Part model, mm, in its own coordinate system. Face numbers are marked on the shaded views. A direction names the side the tool comes from. Coordinates: 2 decimals unless noted, no trailing zeros. Write each loop counter-clockwise with the first axis right and the second up, starting at its lowest first coordinate (ties: lowest second). Pieces come first, ordered by that corner, then holes. Notation, with made-up numbers: M 74,53.25 L 104,53.25 A20 ccw 104,65.25 Z; hole C -14,-10.75 d5. An arc over 180 degrees is marked long. Use a Markdown table: item, result. Add a question column.
Q1. Slice it at C-C on x = -3. Write the cut outline in (y, z), then the cut area to 3 significant figures.
Q2. Wall check: L1, parallel to Z at x = -1, y = 0.75; L2, parallel to Z at x = -2.5, y = 2.6; L3, parallel to X at y = 0.8, z = 6.75. Give the ranges that are in metal, low to high. Write a range as from..to.
Q3. Slice it at D-D on x = 0.75. Write the cut outline in (y, z).
Q4. Mould opens along Z. For the marked faces 3, 4 and 5 say: released by +Z, released by -Z, zero draft, split by the parting line, or undercut.
Q5. Slice it at B-B on y = 2.5. Write the cut outline in (x, z), then the cut area to 3 significant figures.
Q6. Tool access for the marked faces 1 and 2: list every direction of +Z, -Z, +X, -X, +Y, -Y with a clear straight run to the whole face (end or side of a thin tool).
Q7. Pin check, flat tip, straight feed: pin 1 Ø1.8 at (x, z) = (-2.04, 16.65) entering from +Y. Stop position of the tip, or through.
Q8. Slice it at A-A on z = 5.5. Write the cut outline in (x, y), then the cut area to 3 significant figures.
from build123d import *

# Parameters (mm, degrees)
SKETCH1_R           = 1.502144761
SKETCH1_R_2         = 1.500235367
BOSS_EXTRUDE3_DEPTH = 3


with BuildPart() as part:
    # Sketch1 → Boss-Extrude3 (new body)
    with BuildSketch(Plane(origin=(0, 0, 0), x_dir=(1, 0, 0), z_dir=(0, 1, 0))):
        Polygon((-3.272270882, -0.800771607), (-2.124220585, 1.970866991), (-1.964220585, 1.970866991), (-0.816170288, -0.800771607), (1.95546831, 0.34727869), (1.95546831, -17.15272131), (1.95546831, -19.653488119), (-6.043909479, -19.653488119), (-6.043909479, -17.27772131), (-6.043909479, -4.77772131), (-6.043909479, 0.34727869), align=None)
        with Locations((-2.04453169, -6.653488119)):
            Circle(SKETCH1_R, mode=Mode.SUBTRACT)
        with Locations((-2.04453169, -16.653488119)):
            Circle(SKETCH1_R_2, mode=Mode.SUBTRACT)
    extrude(amount=BOSS_EXTRUDE3_DEPTH)


solid = part.part
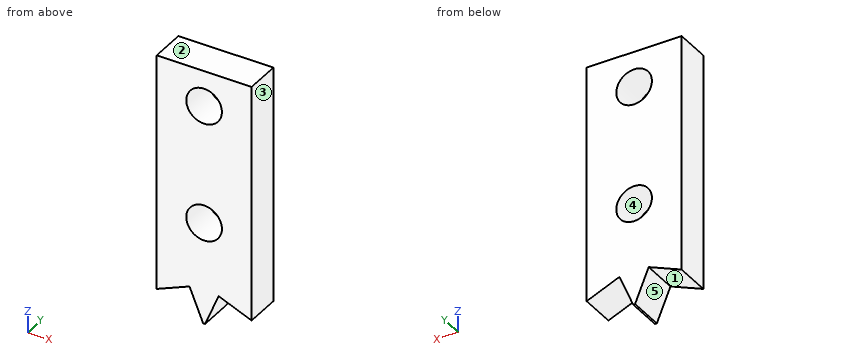
Recorded:
| question | item | result |
|---|---|---|
| 1 | outline | M 0,0.14 L 3,0.14 L 3,5.49 L 0,5.49 Z; M 0,7.81 L 3,7.81 L 3,15.5 L 0,15.5 Z; M 0,17.81 L 3,17.81 L 3,19.65 L 0,19.65 Z |
| 1 | area | 44.6 mm² |
| 2 | L1 | 0.36..5.57, 7.73..15.58, 17.73..19.65 |
| 2 | L2 | -1.06..5.22, 8.08..15.22, 18.08..19.65 |
| 2 | L3 | -6.04..-3.54, -0.55..1.96 |
| 3 | outline | M 0,0.15 L 3,0.15 L 3,19.65 L 0,19.65 Z |
| 4 | face 3 | zero draft |
| 4 | face 4 | undercut |
| 4 | face 5 | released by -Z |
| 5 | outline | M -6.04,-0.35 L -3.27,0.8 L -2.12,-1.97 L -1.96,-1.97 L -0.82,0.8 L 1.96,-0.35 L 1.96,19.65 L -6.04,19.65 Z; hole C -2.04,6.65 d3; hole C -2.04,16.65 d3 |
| 5 | area | 143 mm² |
| 6 | face 1 | -Z, +Y, -Y |
| 6 | face 2 | +Z, +X, -X, +Y, -Y |
| 7 | pin 1 | through |
| 8 | outline | M -6.04,0 L -3.01,0 L -3.01,3 L -6.04,3 Z; M -1.08,0 L 1.96,0 L 1.96,3 L -1.08,3 Z |
| 8 | area | 18.2 mm² |
